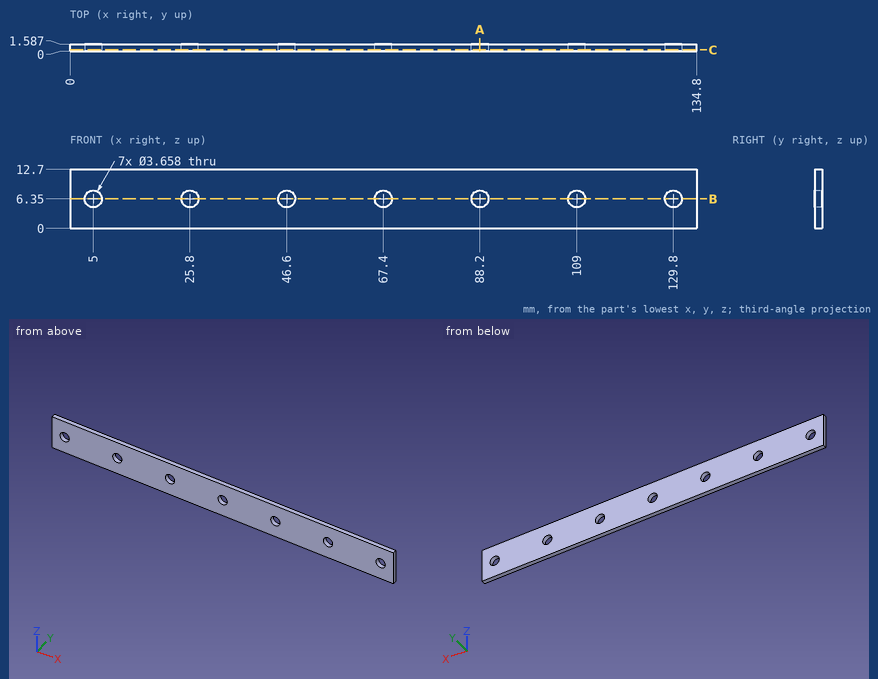
Source: three-view drawing plus pictorial views. Frame: mm from the lowest corner of the part. Coordinates: 2 decimals unless noted, no trailing zeros. Order: outer loops, then holes, each group sorted by start corner. A loop starts at its lowest first (then second) coordinate and runs counter-clockwise, first axis right, second up. Notation, with made-up numbers: (15.25, 74.25) -> (38.25, 74.25) arc R17 cw to (38.25, 86.25) -> close; hole circle Ø9 at (35.25, -32.75). An arc over 180 degrees is marked (long way). Write item = value, one per line.
(1) Pin query (flat end, axial travel): pin 1 Ø2 at (x, z) = (109, 6.35) entering from -Y. Return the tip coordinate at first contact, or that it passes through.
Solved:
pin_1 = through
(2) Cut plane C-C on y = 0.3. Return loops of the section in (x, z).
Solved:
outline = (0, 0) -> (134.8, 0) -> (134.8, 12.7) -> (0, 12.7) -> close; hole circle Ø3.66 at (5, 6.35); hole circle Ø3.66 at (25.8, 6.35); hole circle Ø3.66 at (46.6, 6.35); hole circle Ø3.66 at (67.4, 6.35); hole circle Ø3.66 at (88.2, 6.35); hole circle Ø3.66 at (109, 6.35); hole circle Ø3.66 at (129.8, 6.35)
(3) Cut plane B-B on z = 6.35. Count the separate pieces of the cut face and the enclosed holes in it.
Solved:
separate_pieces = 8
enclosed_holes = 0
(4) Cut plane A-A on x = 88.2. Return loops of the section in (y, z).
Solved:
outline = (0, 0) -> (1.59, 0) -> (1.59, 4.52) -> (0, 4.52) -> close; (0, 8.18) -> (1.59, 8.18) -> (1.59, 12.7) -> (0, 12.7) -> close
(5) Line query: line 1 (Z direction, x = 109, y = 1); line 2 (Z direction, x = 24.5, y = 1.05) (1 decimal). Output: solid intervals per line, ascending.
Solved:
line_1 = 0 to 4.52, 8.18 to 12.7
line_2 = 0 to 5.1, 7.6 to 12.7
